```python
from build123d import *

# Parameters (mm, degrees)
SKETCH1_R          = 0.75
BASE_EXTRUDE_DEPTH = 1


with BuildPart() as part:
    # Sketch1 → Base-Extrude (new body)
    with BuildSketch(Plane.XY):
        with BuildLine():
            Line((-4.385951083, 6.804439308), (-4.385951083, 4.702555787))
            ThreePointArc((-4.385951083, 4.702555787), (-4.449660564, 4.351329273), (-4.632671211, 4.044855677))
            ThreePointArc((-4.632671211, 4.044855677), (0, -6.15), (4.632671211, 4.044855677))
            ThreePointArc((4.632671211, 4.044855677), (4.449660564, 4.351329273), (4.385951083, 4.702555787))
            Line((4.385951083, 4.702555787), (4.385951083, 6.804439308))
            ThreePointArc((4.385951083, 6.804439308), (4.251976487, 7.304439308), (3.885951083, 7.670464712))
            ThreePointArc((3.885951083, 7.670464712), (2.731725093, 8.215797616), (1.503798645, 8.56482806))
            Line((1.503798645, 8.56482806), (1.242331416, 5.576243966))
            ThreePointArc((1.242331416, 5.576243966), (0, -3.8602), (-1.242331416, 5.576243966))
            Line((-1.242331416, 5.576243966), (-1.503798645, 8.56482806))
            ThreePointArc((-1.503798645, 8.56482806), (-2.731725093, 8.215797616), (-3.885951083, 7.670464712))
            ThreePointArc((-3.885951083, 7.670464712), (-4.251976487, 7.304439308), (-4.385951083, 6.804439308))
        make_face()
        with Locations((-2.441520298, 6.834151417)):
            Circle(SKETCH1_R, mode=Mode.SUBTRACT)
        with Locations((2.441520298, 6.834151417)):
            Circle(SKETCH1_R, mode=Mode.SUBTRACT)
    extrude(amount=BASE_EXTRUDE_DEPTH)


solid = part.part
```
The listing builds one solid part. Answer for the finished solid, in the listing's coordinates (mm). A direction names the side the tool comes from. Coordinates: 2 decimals unless noted, no trailing zeros. Write each loop counter-clockwise with the first axis right and the second up, starting at its lowest first coordinate (ties: lowest second). Pieces come first, ordered by that corner, then holes. Notation, with made-up numbers: (41, 54.25) - (60, 54.25) arc R37 ccw to (60, 91.25) - close; hole circle Ø8 at (70, 60). An arc over 180 degrees is marked (long way). Return JSON: item names as keys, results as strings. Group by question number.
Q1. For a pull along X with two mould halves and no side action, classify faces 1 (the cylindrical face through (0.193, -3.856, 0.493)), 2 (the flat face through (2, -4, 0)), 3 (the cylindrical face through (2.75, 8.21, 0.49)) as +X half, -X half, draft (parallel to the pull), parting line (faces both ways), or undercut.
Q2. Which of the six approach directions +Z, -Z, +X, -X, +Y, -Y give full straight-line access (tool end or side, diameter ignored) to faces 4 (the cylindrical face through (-2.6, 6.1, 0.5)), 5 (the flat face through (4.386, 5.7, 0.5)), 6 (the flat face through (1.375, 7.091, 0.493)), 7 (the flat face through (-4.386, 5.8, 0.5))?
Q3. The part is cut by section A-A on y = 0. Write down the section's boundary in (x, z), and give its area (3 significant figures).
Q4. Find the intervals of material crossed by line 1 along Y through (x, z) = (2.25, 0.85); line 2 along Y through (x, z) = (0, 0.5); line 3 along X through (y, z) = (4.5, 0.75), in increasing order. Write a range as [from, to].
Q5. The part is cut by section D-D on z = 0.7. Write down the section's boundary in (x, y), and give its area (3 significant figures).
Q6. The part is cut by section C-C on x = 0. Write down the section's boundary in (y, z).
Q7. The part is cut by section B-B on y = 7. Write down the section's boundary in (x, z).
Evaluation:
{
 "1": {"face 1": "undercut", "face 2": "draft", "face 3": "+X half"},
 "2": {"face 4": "+Z, -Z", "face 5": "+Z, -Z, +X, +Y", "face 6": "+Z, -Z, +Y", "face 7": "+Z, -Z, -X, +Y"},
 "3": {"outline": "(-6.15, 0) - (-4.71, 0) - (-4.71, 1) - (-6.15, 1) - close; (4.71, 0) - (6.15, 0) - (6.15, 1) - (4.71, 1) - close", "area": "2.89 mm2"},
 "4": {"line 1": "y = [-5.72, -3.3], [5.18, 6.11], [7.56, 8.38]", "line 2": "y = [-6.15, -3.86]", "line 3": "x = [-4.41, -3.22], [3.22, 4.41]"},
 "5": {"outline": "(-4.63, 4.04) arc R6.15 ccw (long way) to (4.63, 4.04) arc R1 cw to (4.39, 4.7) - (4.39, 6.8) arc R1 ccw to (3.89, 7.67) arc R7.77 ccw to (1.5, 8.56) - (1.24, 5.58) arc R4.8 cw (long way) to (-1.24, 5.58) - (-1.5, 8.56) arc R7.77 ccw to (-3.89, 7.67) arc R1 ccw to (-4.39, 6.8) - (-4.39, 4.7) arc R1 cw to start; hole circle Ø1.5 at (-2.44, 6.83); hole circle Ø1.5 at (2.44, 6.83)", "area": "58.3 mm2"},
 "6": {"outline": "(-6.15, 0) - (-3.86, 0) - (-3.86, 1) - (-6.15, 1) - close"},
 "7": {"outline": "(-4.37, 0) - (-3.17, 0) - (-3.17, 1) - (-4.37, 1) - close; (-1.71, 0) - (-1.37, 0) - (-1.37, 1) - (-1.71, 1) - close; (1.37, 0) - (1.71, 0) - (1.71, 1) - (1.37, 1) - close; (3.17, 0) - (4.37, 0) - (4.37, 1) - (3.17, 1) - close"}
}
